Check sheet for the modelled part. Datum: model origin and axes. Units: mm. A direction names the side the tool comes from. Round coordinates to 2 decimals unless told otherwise and drop trailing zeros. Loops run counter-clockwise (first coordinate to the right, second up) from the corner with the lowest first, then second, coordinate; pieces in that order, holes last. Notation, with made-up numbers: M 11.25,-22.75 L 37.25,-22.75 A36 ccw 37.25,12.25 Z; hole C -11.75,40 d3. An arc over 180 degrees is marked long. One line per question, with ' | ' between items. Start each with the question number.
(1) Draft check along X on faces 1 (the face through (105, -65, -161)), 2 (the face through (175.49, -120.72, 160.86)), 3 (the face through (-3, -14, -171)), 4 (the face through (-175.72, -120.49, 160.86)). Enter one of: +X half, -X half, draft (parallel to the pull), parting line (faces both ways), or undercut.
(2) Section check A-A (y = -83.5). Record the boundary of the cut face in (x, z), and give its area (3 significant figures).
(3) Section check C-C (z = -24). Record the boundary of the cut face in (x, y), and give its area (3 significant figures).
(4) Thickness scan on probe 1 along Y at (x, z) = (105, -157); probe 2 along Z at (x, y) = (-89, -86); probe 3 along Y at (x, z) = (32, -125). Record the ranges inside material, lowest first. Write a range as [from, to].
(5) Go/stop test with flat-tipped pins: P1, Ø22, axis at x = 20, z = -163, coming from the -Y side; P2, Ø2, axis at x = -126, z = 16, coming from the -Y side. Record where each tip stops, or that it passes through.
(6) Section check D-D (x = -127). Record the boundary of the cut face in (y, z).
(7) Tool access check on faces 5 (the face through (104.133, -68.905, 155.93)), 6 (the face through (114, -125, -161)), 7 (the face through (-3, -6, 151)), 8 (the face through (-50, -71, 161)), 9 (the face through (-54.51, -120.72, 160.86)). Record the directions out of +Z, -Z, +X, -X, +Y, -Y that give a thin tool (end or side, any length) a straight path to the whole face; none if there is none.
(8) Section check B-B (x = 24). Record the boundary of the cut face in (y, z).
```python
from build123d import *

# Parameters (mm, degrees)
SKETCH1_W           = 360
SKETCH1_H           = 342
BOSS_EXTRUDE1_DEPTH = 55
BOSS_EXTRUDE2_DEPTH = 20
SKETCH4_R           = 4
CUT_EXTRUDE2_DEPTH  = 10
FILLET1_R           = 15


with BuildPart() as part:
    # Sketch1 → Boss-Extrude1 (new body)
    with BuildSketch(Plane(origin=(0, 0, 0), x_dir=(1, 0, 0), z_dir=(0, 1, 0))):
        Rectangle(SKETCH1_W, SKETCH1_H)
    extrude(amount=BOSS_EXTRUDE1_DEPTH)

    # Sketch2 → Boss-Extrude2 (add)
    with BuildSketch(Plane.XY.offset(171)):
        Polygon((180, 0), (0, 0), (0, -15), (50, -15), (50, -125), (180, -125), align=None)
        Polygon((0, 0), (-180, 0), (-180, -125), (-50, -125), (-50, -15), (0, -15), align=None)
    boss_extrude2 = extrude(amount=-BOSS_EXTRUDE2_DEPTH)

    # Sketch4 → Cut-Extrude2 (cut)
    with BuildSketch(Plane.XY.offset(151)):
        with Locations((105, -65)):
            Circle(SKETCH4_R)
        with Locations(Location((-105, -65, 0), (0, 0, 180))):
            Circle(SKETCH4_R)
    cut_extrude2 = extrude(amount=CUT_EXTRUDE2_DEPTH, mode=Mode.SUBTRACT)

    # Fillet1
    fillet1_edges = [part.edges().sort_by_distance(p)[0] for p in [
        (180, -125, 161),
        (50, -125, 161),
        (50, -15, 161),
        (-50, -15, 161),
        (-50, -125, 161),
        (-180, -125, 161),
    ]]
    fillet(fillet1_edges, radius=FILLET1_R)

    # Mirror1: Boss-Extrude2, Cut-Extrude2 across plane
    add(boss_extrude2.mirror(Plane.XY))
    add(cut_extrude2.mirror(Plane.XY), mode=Mode.SUBTRACT)


solid = part.part
```
The answers:
1) face 1: undercut | face 2: +X half | face 3: draft | face 4: -X half
2) outline: M -180,-171 L -50,-171 L -50,-151 L -180,-151 Z; M -180,151 L -50,151 L -50,171 L -180,171 Z; M 50,-171 L 180,-171 L 180,-151 L 50,-151 Z; M 50,151 L 180,151 L 180,171 L 50,171 Z | area: 10,400 mm²
3) outline: M -180,0 L 180,0 L 180,55 L -180,55 Z | area: 19,800 mm²
4) probe 1: [-125, -69], [-61, 55] | probe 2: [-171, -151], [151, 171] | probe 3: [0, 55]
5) P1: y = -15 | P2: y = 0
6) outline: M -125,-171 L 55,-171 L 55,171 L -125,171 L -125,151 L 0,151 L 0,-151 L -125,-151 Z
7) face 5: none | face 6: +Z, -Z, +X, -X, -Y | face 7: +X, -X, -Y | face 8: +Z, -Z, -Y | face 9: +Z, -Y
8) outline: M -15,-171 L 55,-171 L 55,171 L -15,171 L -15,151 L 0,151 L 0,-151 L -15,-151 Z
